Drawing for the job (mm, zero at the part's lowest x, y, z). A direction names the side the tool comes from. Give positions to 0.01 mm unless a question says otherwise; leave off trailing zeros. Order: outer loops, then holes, each group sorted by start corner. A loop starts at its lowest first (then second) coordinate and runs counter-clockwise, first axis right, second up. Notation, with made-up numbers: (27, -29.5) - (56, -29.5) arc R24 cw to (56, -11.5) - close; hole circle Ø6 at (57, 43.5). An arc over 180 degrees is marked (long way). One line per item, written item: value.
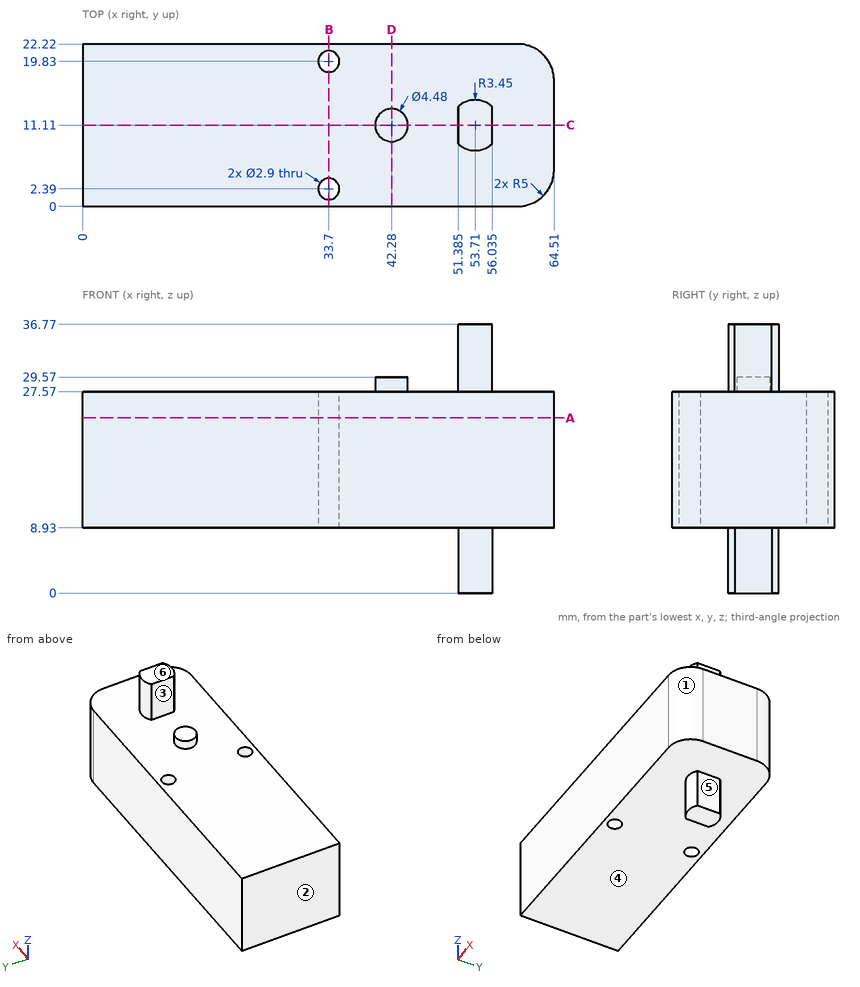
1) Pin check, flat tips, straight feed: pin 1 (1 mm diameter, centred on x = 26.5, y = 7.5, fed in from +Z); pin 2 (3 mm diameter, centred on x = 44.5, z = 17, fed in from -Y); pin 3 (2.5 mm diameter, centred on y = 11, z = 4, fed in from -X) (3 decimals); pin 4 (1.3 mm diameter, centred on x = 42, y = 12, fed in from +Z). Stop position of each tip, or through.
Outcome:
pin 1: stops at z = 27.57
pin 2: stops at y = 0
pin 3: stops at x = 51.385
pin 4: stops at z = 29.57
2) Cut at A-A, the plane z = 24. Give the cut face in (x, y).
Outcome:
outline: (0, 0) - (59.51, 0) arc R5 ccw to (64.51, 5) - (64.51, 17.22) arc R5 ccw to (59.51, 22.22) - (0, 22.22) - close; hole circle Ø2.9 at (33.7, 2.39); hole circle Ø2.9 at (33.7, 19.83)
3) Drill centre lines: line 1 along Y through (x, z) = (33.7, 15.5); line 2 along Y through (x, z) = (33, 17); line 3 along Z through (x, y) = (26.5, 2.5). Where is each one in solid material? Low to high. Write a range as from..to.
Outcome:
line 1: y = 0..0.94, 3.84..18.38, 21.28..22.22
line 2: y = 0..1.12, 3.66..18.56, 21.1..22.22
line 3: z = 8.93..27.57
4) Cut at D-D, the plane x = 42.28. Give the cut face in (y, z), then the cut area to 3 significant figures.
Outcome:
outline: (0, 8.93) - (22.22, 8.93) - (22.22, 27.57) - (13.35, 27.57) - (13.35, 29.57) - (8.87, 29.57) - (8.87, 27.57) - (0, 27.57) - close
area: 423 mm^2
5) Mould opens along X. For the marked faces 1, 2, 3 and 4 say: released by +X, released by -X, zero draft, split by the parting line, or undercut.
Outcome:
face 1: released by +X
face 2: released by -X
face 3: undercut
face 4: zero draft
6) Cut at B-B, the plane x = 33.7. Give the cut face in (y, z).
Outcome:
outline: (0, 8.93) - (0.94, 8.93) - (0.94, 27.57) - (0, 27.57) - close; (3.84, 8.93) - (18.38, 8.93) - (18.38, 27.57) - (3.84, 27.57) - close; (21.28, 8.93) - (22.22, 8.93) - (22.22, 27.57) - (21.28, 27.57) - close
7) Which spindle directions (+Z, -Z, +X, -X, +Y, -Y) get a long thin tool onto all of the face, cutting with end or side? Do the marked faces 5 and 6. Say none if no direction does.
Outcome:
face 5: -Z, +X, +Y, -Y
face 6: +Z, +X, -X, +Y, -Y
8) Cut at C-C, the plane y = 11.11. Give the cut face in (x, z) (3 decimals).
Outcome:
outline: (0, 8.93) - (51.385, 8.93) - (51.385, 0) - (56.035, 0) - (56.035, 8.93) - (64.51, 8.93) - (64.51, 27.57) - (56.035, 27.57) - (56.035, 36.77) - (51.385, 36.77) - (51.385, 27.57) - (44.52, 27.57) - (44.52, 29.57) - (40.04, 29.57) - (40.04, 27.57) - (0, 27.57) - close
